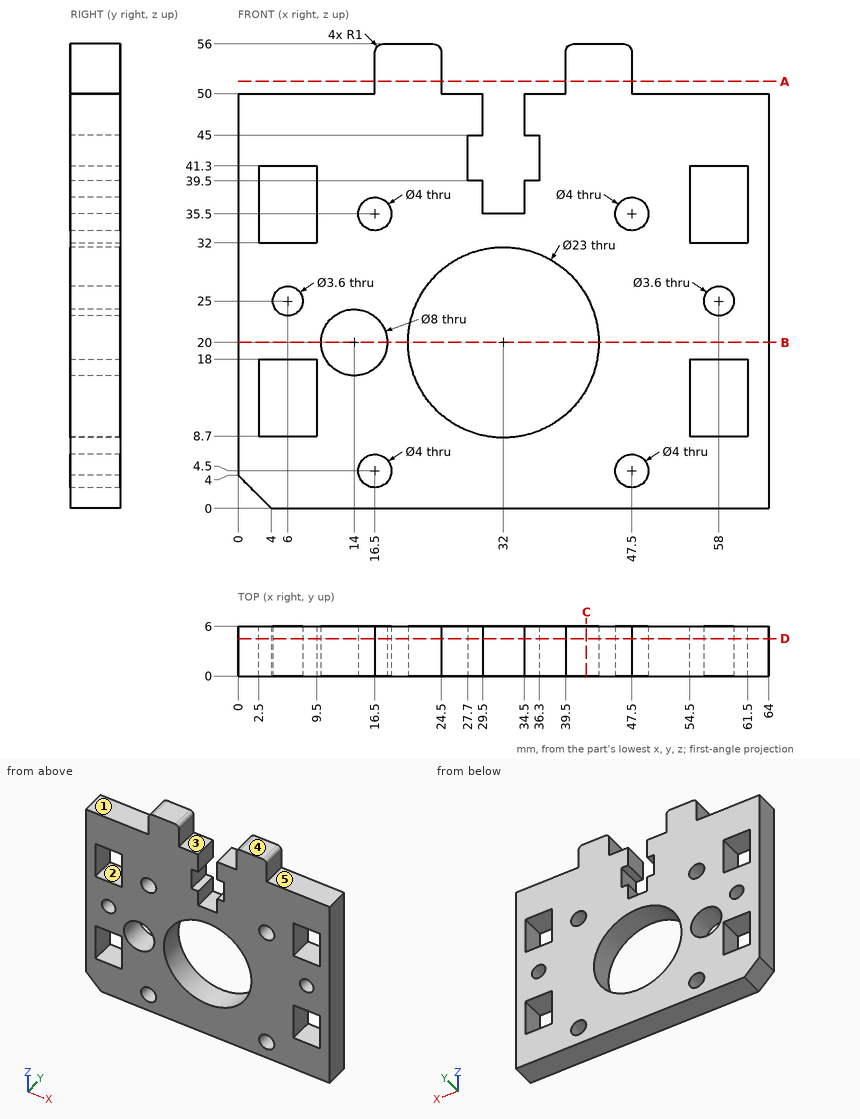
Check sheet for the drawn part. Datum: minimum x, y, z corner. Units: mm. A direction names the side the tool comes from. Round coordinates to 2 decimals unless told otherwise and drop trailing zeros. Order: outer loops, then holes, each group sorted by start corner. A loop starts at its lowest first (then second) coordinate and runs counter-clockwise, first axis right, second up. Notation, with made-up numbers: M 59.5,25.5 L 67.5,25.5 A32 ccw 67.5,61.5 Z; hole C 53.5,12 d1. An arc over 180 degrees is marked long. Write each question's results on one line, items separated by ' | '. Start each with the question number.
1. Cross-section at A-A on z = 51.5. Record the boundary of the cut face in (x, y), plus the area to 3 significant figures.
2. Cross-section at D-D on y = 4.5. Give the number of separate pieces and of enclosed holes in the cut face, plus the area to 3 significant figures.
3. Cross-section at B-B on z = 20. Record the boundary of the cut face in (x, y), plus the area to 3 significant figures.
4. Go/stop test with flat-tipped pins: P1, Ø2, axis at y = 0.5, z = 34.5, coming from the -X side; P2, Ø1.4, axis at x = 36, y = 2, coming from the +Z side; P3, Ø1.5, axis at y = 4.5, z = 53.5, coming from the +X side; P4, Ø2.5, axis at x = 47.5, z = 35.5, coming from the +Y side. Record where each tip stops, or that it passes through.
5. Material ranges on L1, parallel to X at y = 1.65, z = 20; L2, parallel to X at y = 1.3, z = 4.5; L3, parallel to Z at x = 58, y = 4.5, recorded low to high. Write a range as from..to.
6. Set-up check for the marked faces 1, 2, 3, 4 and 5: record each of +Z, -Z, +X, -X, +Y, -Y from which the full face is reachable in a straight line by a thin tool's end or side.
7. Cross-section at C-C on x = 42. Record the boundary of the cut face in (y, z).
Resolved:
1) outline: M 16.5,0 L 24.5,0 L 24.5,6 L 16.5,6 Z; M 39.5,0 L 47.5,0 L 47.5,6 L 39.5,6 Z | area: 96.0 mm2
2) separate pieces: 1 | enclosed holes: 12 | area: 2,400 mm2
3) outline: M 0,0 L 10,0 L 10,6 L 0,6 Z; M 18,0 L 20.5,0 L 20.5,6 L 18,6 Z; M 43.5,0 L 64,0 L 64,6 L 43.5,6 Z | area: 198 mm2
4) P1: x = 0 | P2: z = 50 | P3: x = 47.5 | P4: through
5) L1: 0..10, 18..20.5, 43.5..64 | L2: 0..14.5, 18.5..45.5, 49.5..64 | L3: 0..8.7, 18..23.2, 26.8..32, 41.3..50
6) face 1: +Z, -X, +Y, -Y | face 2: +Y, -Y | face 3: +Z, +Y, -Y | face 4: +Z, +X, -X, +Y, -Y | face 5: +Z, +X, +Y, -Y
7) outline: M 0,0 L 6,0 L 6,14.32 L 0,14.32 Z; M 0,25.68 L 6,25.68 L 6,56 L 0,56 Z
